from build123d import *

# Parameters (mm, degrees)
SKETCH1_R           = 20.6
BOSS_EXTRUDE1_DEPTH = 2
SKETCH2_R           = 5.15
CUT_EXTRUDE1_DEPTH  = 3
SKETCH3_R           = 6.5
CUT_EXTRUDE2_DEPTH  = 2
BOSS_EXTRUDE4_DEPTH = 22
FILLET2_R           = 5


with BuildPart() as part:
    # Sketch1 → Boss-Extrude1 (new body)
    with BuildSketch(Plane(origin=(0, 0, 0), x_dir=(1, 0, 0), z_dir=(0, 1, 0))):
        with Locations(Location((0, 0, 0), (0, 0, 270))):
            Circle(SKETCH1_R)
    extrude(amount=BOSS_EXTRUDE1_DEPTH)

    # Sketch2 → Cut-Extrude1 (cut)
    with BuildSketch(Plane(origin=(0, 2, 0), x_dir=(1, 0, 0), z_dir=(0, 1, 0))):
        with Locations(Location((0, 0, 0), (0, 0, 270))):
            Circle(SKETCH2_R)
    extrude(amount=-CUT_EXTRUDE1_DEPTH, mode=Mode.SUBTRACT)

    # Sketch3 → Cut-Extrude2 (cut)
    with BuildSketch(Plane(origin=(0, 2, 0), x_dir=(1, 0, 0), z_dir=(0, 1, 0))):
        with Locations(Location((0, 13, 0), (0, 0, 270))):
            Circle(SKETCH3_R)
    extrude(amount=-CUT_EXTRUDE2_DEPTH, mode=Mode.SUBTRACT)

    # Sketch4 → Boss-Extrude4 (add)
    with BuildSketch(Plane(origin=(0, 2, 0), x_dir=(1, 0, 0), z_dir=(0, 1, 0))):
        with BuildLine():
            Line((-16.743954133, 12), (-3.5, 5.5))
            Line((-3.5, 5.5), (3.5, 5.5))
            Line((3.5, 5.5), (16.743954133, 12))
            ThreePointArc((16.743954133, 12), (13.279606143, 15.748398671), (9, 18.529975715))
            ThreePointArc((9, 18.529975715), (0, 6.042759079), (-9, 18.529975715))
            ThreePointArc((-9, 18.529975715), (-13.279606143, 15.748398671), (-16.743954133, 12))
        make_face()
    extrude(amount=BOSS_EXTRUDE4_DEPTH)

    # Fillet2
    # the kernel refuses this fillet: 5 mm, written as the material it takes off along each edge
    with BuildSketch(Plane(origin=(-16.743954133, 2, -12), x_dir=(0.7333047678367514, 0, -0.6799000790321236), z_dir=(0, 1, 0))) as fillet2_piece_1:
        with BuildLine():
            CenterArc((7.239333023, -4.898998289), FILLET2_R, 78.464118396, 122.558704485)
            Line((2.572145012, -6.692697281), (0, 0))
            ThreePointArc((0, 0), (4.11962045, 0.416127048), (8.239240899, 0))
        make_face()
    extrude(amount=42.598102248, mode=Mode.SUBTRACT)
    with BuildSketch(Plane(origin=(16.743954133, 2, -12), x_dir=(-0.7333047678367518, 0, -0.6799000790321232), z_dir=(0, 1, 0))) as fillet2_piece_2:
        with BuildLine():
            CenterArc((7.239333023, 4.898998289), FILLET2_R, 158.97717712, 122.558704485)
            Line((2.572145012, 6.692697281), (0, 0))
            ThreePointArc((0, 0), (4.11962045, -0.416127048), (8.239240899, 0))
        make_face()
    extrude(amount=42.598102248, mode=Mode.SUBTRACT)


solid = part.part
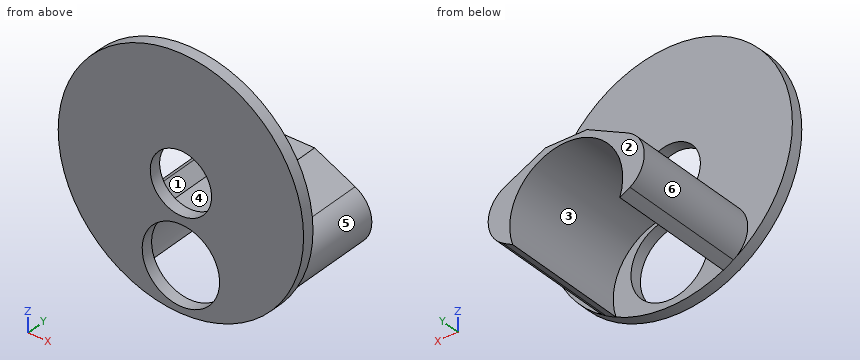
Build history of the part. All positions in model axes, mm. Face numbers are marked on the shaded views. A direction names the side the tool comes from. Coordinates: 2 decimals unless noted, no trailing zeros. Write each loop counter-clockwise with the first axis right and the second up, starting at its lowest first coordinate (ties: lowest second). Pieces come first, ordered by that corner, then holes.
(1) Mould opens along X. For the marked faces 1, 2 and 3 say: pulls with the +X half, pulls with the -X half, needs draft (parallel to the pull), parting line crosses it, or undercut.
(2) Cut at D-D on z = -13. List the corners of the cut face in (x, y).
(3) 3-axis set-ups, long thin cutter, end or side, ignore diameter. For the marked faces 4, 5 and 6: which of +Z, -Z, +X, -X, +Y, -Y reach the whole face in a straight line?
(4) Cut at C-C on y = 13.25. List the corners of the cut face in (x, z).
(5) Pin check, flat tips, straight feed: pin 1 Ø4.5 at (x, z) = (0.5, -11) entering from +Y; pin 2 Ø5 at (x, y) = (-2, 13) entering from -Z; pin 3 Ø4 at (y, z) = (9, -14) entering from -X; pin 4 Ø5 at (x, y) = (0.5, 8.5) entering from -Z. Stop position of each tip, or through.
(6) Drill centre lines: line 1 (X direction, y = 0.45, z = 0); line 2 (Y direction, x = 4.5, z = 14.5); line 3 (X direction, y = 16.5, z = -17). Where is each one in solid material? Low to high.
(7) Cut at A-A on x = 0. List the corners of the cut face in (y, z).
(8) Cut at B-B on z = 0. List the corners of the cut face in (x, y).
Working result:
1. face 1: pulls with the -X half
1. face 2: needs draft
1. face 3: undercut
2. outline: (-15.98, 0) - (-6.5, 0) - (-6.5, 2) - (-9.14, 2) - (-9.14, 24) - (-13.09, 24) - (-13.09, 2) - (-15.98, 2) - close; (6.5, 0) - (15.98, 0) - (15.98, 2) - (13.09, 2) - (13.09, 24) - (9.14, 24) - (9.14, 2) - (6.5, 2) - close
3. face 4: +Z, +X, -X, +Y
3. face 5: +X, +Y
3. face 6: -X, +Y
4. outline: (-10.7, -17.6) arc R20.6 ccw to (-9, -18.53) arc R9.49 cw (long way) to (9, -18.53) arc R20.6 ccw to (10.7, -17.6) arc R5 ccw to (10.31, -8.84) - (3.5, -5.5) - (-3.5, -5.5) - (-10.31, -8.84) arc R5 ccw to start
5. pin 1: passes through
5. pin 2: stops at z = -7.18
5. pin 3: stops at x = -13.1
5. pin 4: stops at z = -6.53
6. line 1: x = -20.6 to -5.15, 5.15 to 20.6
6. line 2: y = 0 to 2
6. line 3: x = -11.5 to -9.37, 9.37 to 11.5
7. outline: (0, -20.6) - (2, -20.6) - (2, -19.5) - (0, -19.5) - close; (0, -6.5) - (2, -6.5) - (2, -6.04) - (24, -6.04) - (24, -5.5) - (2, -5.5) - (2, -5.15) - (0, -5.15) - close; (0, 5.15) - (2, 5.15) - (2, 20.6) - (0, 20.6) - close
8. outline: (-20.6, 0) - (-5.15, 0) - (-5.15, 2) - (-20.6, 2) - close; (5.15, 0) - (20.6, 0) - (20.6, 2) - (5.15, 2) - close
